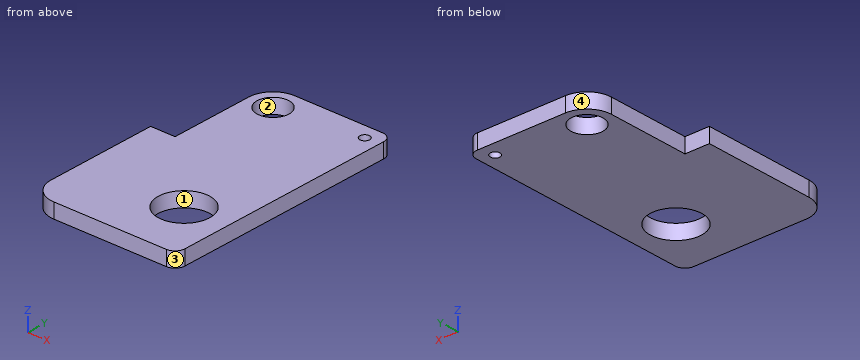
Autodesk Inventor part; units mm, degrees
ref_plane "YZ Plane" through (0, 0, 0) normal (1, 0, 0) x (0, 1, 0)
ref_plane "XZ Plane" through (0, 0, 0) normal (0, 1, 0) x (-1, 0, 0)
ref_plane "XY Plane" through (0, 0, 0) normal (0, 0, 1) x (1, 0, 0)
sketch "Sketch1" plane through (0, 0, 0) normal (0, 0, 1) x (1, 0, 0)
  line L0 (0, 0) -> (10, 0)
  line L1 (10, 0) -> (10, 10)
  line L2 (10, 10) -> (0, 10)
  line L3 (0, 10) -> (0, 0)
  line L4 (10, 10) -> (25, 10)
  line L5 (25, 10) -> (25, 4)
  line L6 (25, 4) -> (10, 4)
  line L7 (10, 4) -> (10, 10)
  line L8 (10, 0) -> (0, 0)
  line L9 (0, 0) -> (0, -40)
  line L10 (0, -40) -> (10, -40)
  line L11 (10, -40) -> (10, 0)
  line L12 (0, -40) -> (-5, -40)
  line L13 (-5, -40) -> (-5, -12)
  line L14 (-5, -12) -> (0, -12)
  line L15 (0, -12) -> (0, -40)
  line L16 (10, 4) -> (25, 4)
  line L17 (25, 4) -> (25, -40)
  line L18 (25, -40) -> (10, -40)
  line L19 (10, -40) -> (10, 4)
  dimension "d0" = 10
  dimension "d2" = 15
  dimension "d3" = 6
  dimension "d5" = 28
  dimension "d6" = 5
  dimension "d7" = 10
  dimension "d30" = 22
extrude "Extrusion1" add sketch "Sketch1" along normal blind 3
fillet "Fillet1" radius 5 1 edges at (0, 10, 1.5)
fillet "Fillet2" radius 5 1 edges at (-5, -40, 1.5)
fillet "Fillet3" [suppressed]
fillet "Fillet4" [suppressed]
sketch "Sketch2" plane through (0, 0, 3) normal (0, 0, 1) x (1, 0, 0)
  arc A0 (22, 4) -> (22, 10) centre (22, 7) ccw
  point P0 (0, 0)
hole "Hole1" at (22, 7, 3) direction (0, 0, -1) diameter 2 end through all
sketch "Sketch3" plane through (0, 0, 3) normal (0, 0, 1) x (1, 0, 0)
  line L0 (25, 10) -> (5, 10)
  line L1 (0, 5) -> (0, -12)
  point P0 (0, 0)
  point P1 (5, 5)
  point P2 (22, 10)
  dimension "d20" = 5
  dimension "d31" = 5
hole "Hole2" at (5, 5, 3) direction (0, 0, -1) diameter 6.5 end through all
fillet "Fillet6" radius 2 2 edges at (25, 10, 1.5) (25, -40, 1.5)
sketch "Sketch4" plane through (0, 0, 3) normal (0, 0, 1) x (1, 0, 0)
  line L0 (25, -38) -> (25, 8)
  line L1 (0, -40) -> (23, -40)
  point P0 (0, 0)
  point P1 (16, -28)
  dimension "d33" = 9
  dimension "d34" = 12
hole "Hole3" at (16, -28, 3) direction (0, 0, -1) diameter 10.5 end through all
properties part number "Selection_Lever 1" material "Nylon 6/6"
The model under review builds one solid part; all positions refer to its coordinate system, in mm. Face numbers are marked on the shaded views. Give positions to 0.01 mm unless a question says otherwise; leave off trailing zeros. Write each loop counter-clockwise with the first axis right and the second up, starting at its lowest first coordinate (ties: lowest second). Pieces come first, ordered by that corner, then holes. Notation, with made-up numbers: M 59,-25 L 104,-25 A36 cw 104,10 Z; hole C 40,19.25 d9. An arc over 180 degrees is marked long. Answer in a Markdown table with one row per item.
Item 1: Add section D-D on y = 7. Give the boundary of the cut face in (x, z), plus the area to 3 significant figures.
Check sheet entries:
| item | result |
|---|---|
| outline | M 0.42,0 L 2.44,0 L 2.44,3 L 0.42,3 Z; M 7.56,0 L 21,0 L 21,3 L 7.56,3 Z; M 23,0 L 25,0 L 25,3 L 23,3 Z |
| area | 52.4 mm2 |
Item 2: Draft analysis for pull direction Y (two halves, no side actions). For the marked faces 1, 2, 3 and 4, state which applies: +Y half, -Y half, draft (parallel to the pull), parting line (faces both ways), or undercut.
Check sheet entries:
| item | result |
|---|---|
| face 1 | undercut |
| face 2 | undercut |
| face 3 | -Y half |
| face 4 | +Y half |
Item 3: For P1, Ø1, axis at x = 4.5, z = 2.5, coming from the +Y side; P2, Ø1.5, axis at y = -10.5, z = 2.5, coming from the -X side, all flat-tipped, find the tip position at first contact; note any pin that passes through.
Check sheet entries:
| item | result |
|---|---|
| P1 | y = 10 |
| P2 | x = 0 |
Item 4: For line 1 along X through (y, z) = (5, 2.15); line 2 along Y through (x, z) = (22, 1.9); line 3 along X through (y, z) = (1.5, 2.2), list the stretches that pass through material, from the lowest coordinate up.
Check sheet entries:
| item | result |
|---|---|
| line 1 | 0 to 1.75, 8.25 to 25 |
| line 2 | -40 to 6, 8 to 10 |
| line 3 | 0 to 25 |
Item 5: Add section B-B on z = 0.6. Give the boundary of the cut face in (x, y), plus the area to 3 significant figures.
Check sheet entries:
| item | result |
|---|---|
| outline | M -5,-35 A5 ccw 0,-40 L 23,-40 A2 ccw 25,-38 L 25,8 A2 ccw 23,10 L 5,10 A5 ccw 0,5 L 0,-12 L -5,-12 Z; hole C 5,5 d6.5; hole C 16,-28 d10.5; hole C 22,7 d2 |
| area | 1,250 mm2 |
Item 6: Add section A-A on y = -28. Give the boundary of the cut face in (x, z), plus the area to 3 significant figures.
Check sheet entries:
| item | result |
|---|---|
| outline | M -5,0 L 10.75,0 L 10.75,3 L -5,3 Z; M 21.25,0 L 25,0 L 25,3 L 21.25,3 Z |
| area | 58.5 mm2 |
Item 7: Add section C-C on x = 16. Give the boundary of the cut face in (y, z).
Check sheet entries:
| item | result |
|---|---|
| outline | M -40,0 L -33.25,0 L -33.25,3 L -40,3 Z; M -22.75,0 L 10,0 L 10,3 L -22.75,3 Z |
